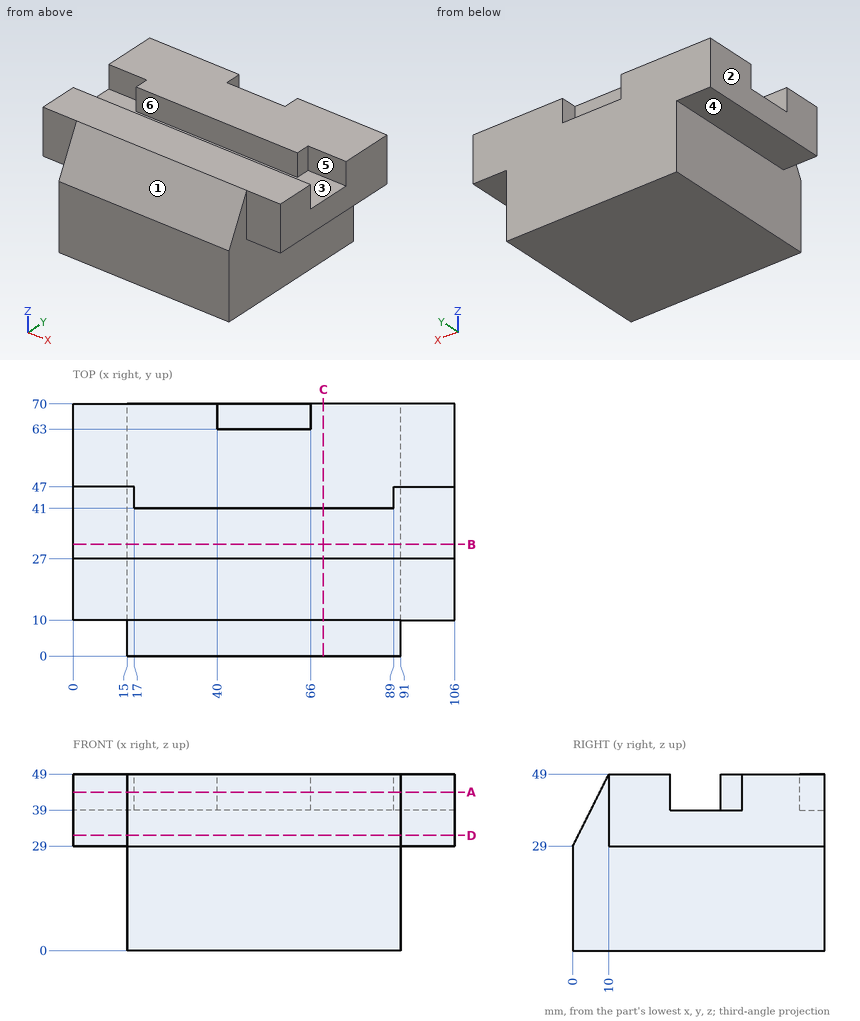
Here's the drawing with two shaded views (mm, measured from the low corner). I have some questions. A direction names the side the tool comes from. Give positions to 0.01 mm unless a question says otherwise; leave off trailing zeros. Loops run counter-clockwise (first coordinate to the right, second up) from the corner with the lowest first, then second, coordinate; pieces in that order, holes last. Notation, with made-up numbers: M 60,81 L 108,81 A24 cw 108,92 Z; hole C -8,55.5 d8. An arc over 180 degrees is marked long. Use one line per item in the form item = value. Start each with the question number.
(1) Please list where these lines run through material, in increasing order: line 1 (Y direction, x = 101.5, z = 45.5); line 2 (Z direction, x = 11, y = 46); line 3 (Z direction, x = 68, y = 37).
(2) Thinking about a two-plate mould opening in Y: for the marked faces 1, 2 and 3, which applies, released by +Y, released by -Y, zero draft, split by the parting line, or undercut?
(3) I'm going to push flat-ended pins straight in: P1, Ø8, axis at x = 51.5, z = 45, coming from the -Y side; P2, Ø8, axis at x = 49, z = 44.5, coming from the +Y side; P3, Ø16.5, axis at x = 102, y = 39, coming from the -Z side. Where does each tip first touch, or does it pass through?
(4) I want a section at C-C, the plane x = 69.5. Write out the boundary of the cut face in (y, z), and give its area (3 significant figures).
(5) I want a section at A-A, the plane z = 44. Write out the boundary of the cut face in (x, y), and give its area (3 significant figures).
(6) I want a section at D-D, the plane z = 32. Write out the boundary of the cut face in (x, y), and give its area (3 significant figures).
(7) On a 3-axis mill with a long thin cutter (end or side, diameter ignored), from which of +Z, -Z, +X, -X, +Y, -Y can I reach the whole of each face in a straight line? I mean the marked faces 4, 5 and 6. Say none if no direction works.
(8) I want a section at B-B, the plane y = 31. Write out the boundary of the cut face in (x, z).
Worked out:
q1.line_1 = 10 to 27, 47 to 70
q1.line_2 = 29 to 39
q1.line_3 = 0 to 39
q2.face_1 = released by -Y
q2.face_2 = zero draft
q2.face_3 = undercut
q3.P1 = 6
q3.P2 = 63
q3.P3 = 29
q4.outline = M 0,0 L 70,0 L 70,49 L 41,49 L 41,39 L 27,39 L 27,49 L 10,49 L 0,29 Z
q4.area = 3,190 mm²
q5.outline = M 0,10 L 15,10 L 15,7.5 L 91,7.5 L 91,10 L 106,10 L 106,27 L 0,27 Z; M 0,47 L 17,47 L 17,41 L 89,41 L 89,47 L 106,47 L 106,70 L 66,70 L 66,63 L 40,63 L 40,70 L 0,70 Z
q5.area = 4,680 mm²
q6.outline = M 0,10 L 15,10 L 15,1.5 L 91,1.5 L 91,10 L 106,10 L 106,70 L 0,70 Z
q6.area = 7,010 mm²
q7.face_4 = -Z, -X, +Y, -Y
q7.face_5 = +Z, +X
q7.face_6 = +Z, +X, -X
q8.outline = M 0,29 L 15,29 L 15,0 L 91,0 L 91,29 L 106,29 L 106,39 L 0,39 Z
